from build123d import *

# Parameters (mm, degrees)
BOX_W             = 8
BOX_H             = 1
BOX_DEPTH         = 4
TUBE016_R         = 4
TUBE016_R_2       = 2.6
TUBE016_DEPTH     = 1
BOX067_W          = 8
BOX067_H          = 1
BOX067_DEPTH      = 4
TUBE019_R         = 4
TUBE019_R_2       = 2.6
TUBE019_DEPTH     = 1
BOX051_W          = 17
BOX051_H          = 8
BOX051_DEPTH      = 2
CYLINDER093_R     = 1.6
CYLINDER093_DEPTH = 8
CYLINDER094_R     = 1.6
CYLINDER094_DEPTH = 8
CYLINDER095_R     = 1.6
CYLINDER095_DEPTH = 8
CYLINDER092_R     = 1.6
CYLINDER092_DEPTH = 8
CYLINDER084_R     = 3.5
CYLINDER084_DEPTH = 2.5
BOX033_W          = 29.5
BOX033_H          = 2.5
BOX033_DEPTH      = 6
CYLINDER082_R     = 3.5
CYLINDER082_DEPTH = 2.5
BOX021_W          = 29.5
BOX021_H          = 2.5
BOX021_DEPTH      = 6
BOX022_W          = 29.5
BOX022_H          = 26
BOX022_DEPTH      = 2
BOX029_W          = 2.5
BOX029_H          = 21
BOX029_DEPTH      = 6
BOX036_W          = 2.5
BOX036_H          = 21
BOX036_DEPTH      = 6
FILLET006_R       = 2
FILLET007_R       = 2


with BuildPart() as cube:
    # Box → Box (new body)
    with BuildSketch(Plane(origin=(-4, -7, 0), x_dir=(1, 0, 0), z_dir=(0, 0, 1))):
        with Locations((4, 0.5)):
            Rectangle(BOX_W, BOX_H)
    extrude(amount=BOX_DEPTH)


with BuildPart() as cut068:
    # Tube016 → Tube016 (new body)
    with BuildSketch(Plane.XZ.offset(6)):
        Circle(TUBE016_R)
        Circle(TUBE016_R_2, mode=Mode.SUBTRACT)
    extrude(amount=TUBE016_DEPTH)

    # Cut068: cut Cube
    add(cube.part, mode=Mode.SUBTRACT)


with BuildPart() as cube067:
    # Box067 → Box067 (new body)
    with BuildSketch(Plane(origin=(-4, -34, 0), x_dir=(1, 0, 0), z_dir=(0, 0, 1))):
        with Locations((4, 0.5)):
            Rectangle(BOX067_W, BOX067_H)
    extrude(amount=BOX067_DEPTH)


with BuildPart() as cut071:
    # Tube019 → Tube019 (new body)
    with BuildSketch(Plane.XZ.offset(33)):
        Circle(TUBE019_R)
        Circle(TUBE019_R_2, mode=Mode.SUBTRACT)
    extrude(amount=TUBE019_DEPTH)

    # Cut071: cut Cube067
    add(cube067.part, mode=Mode.SUBTRACT)


with BuildPart() as cube051:
    # Box051 → Box051 (new body)
    with BuildSketch(Plane(origin=(-8.5, -49, -8), x_dir=(1, 0, 0), z_dir=(0, 0, 1))):
        with Locations((8.5, 4)):
            Rectangle(BOX051_W, BOX051_H)
    extrude(amount=BOX051_DEPTH)


with BuildPart() as cylinder093:
    # Cylinder093 → Cylinder093 (new body)
    with BuildSketch(Plane(origin=(-10, -55, 0), x_dir=(1, 0, 0), z_dir=(0, 0, 1))):
        Circle(CYLINDER093_R)
    extrude(amount=CYLINDER093_DEPTH)


with BuildPart() as cylinder094:
    # Cylinder094 → Cylinder094 (new body)
    with BuildSketch(Plane(origin=(12.5, -36, 0), x_dir=(1, 0, 0), z_dir=(0, 0, 1))):
        Circle(CYLINDER094_R)
    extrude(amount=CYLINDER094_DEPTH)


with BuildPart() as cylinder095:
    # Cylinder095 → Cylinder095 (new body)
    with BuildSketch(Plane(origin=(12.5, -55, 0), x_dir=(1, 0, 0), z_dir=(0, 0, 1))):
        Circle(CYLINDER095_R)
    extrude(amount=CYLINDER095_DEPTH)


with BuildPart() as fusion059:
    # Cylinder092 → Cylinder092 (new body)
    with BuildSketch(Plane(origin=(-10, -36, 0), x_dir=(1, 0, 0), z_dir=(0, 0, 1))):
        Circle(CYLINDER092_R)
    extrude(amount=CYLINDER092_DEPTH)

    # Fusion058: union Cylinder093, Cylinder094, Cylinder095
    add(cylinder093.part)
    add(cylinder094.part)
    add(cylinder095.part)


with BuildPart() as fusion059_1:
    # Fusion058 placement: moved
    add(fusion059.part.moved(Location((0, 0, -8))))

    # Fusion059: union Cube051
    add(cube051.part)


with BuildPart() as cylinder084:
    # Cylinder084 → Cylinder084 (new body)
    with BuildSketch(Plane.XZ.offset(55.5)):
        Circle(CYLINDER084_R)
    extrude(amount=CYLINDER084_DEPTH)


with BuildPart() as cut038:
    # Box033 → Box033 (new body)
    with BuildSketch(Plane(origin=(-13.5, -58, -6), x_dir=(1, 0, 0), z_dir=(0, 0, 1))):
        with Locations((14.75, 1.25)):
            Rectangle(BOX033_W, BOX033_H)
    extrude(amount=BOX033_DEPTH)

    # Cut038: cut Cylinder084
    add(cylinder084.part, mode=Mode.SUBTRACT)


with BuildPart() as cut038_1:
    # Cut038 placement: moved
    add(cut038.part.moved(Location((0, 23, 0))))


with BuildPart() as cylinder082:
    # Cylinder082 → Cylinder082 (new body)
    with BuildSketch(Plane.XZ.offset(55.5)):
        Circle(CYLINDER082_R)
    extrude(amount=CYLINDER082_DEPTH)


with BuildPart() as cut036:
    # Box021 → Box021 (new body)
    with BuildSketch(Plane(origin=(-13.5, -58, -6), x_dir=(1, 0, 0), z_dir=(0, 0, 1))):
        with Locations((14.75, 1.25)):
            Rectangle(BOX021_W, BOX021_H)
    extrude(amount=BOX021_DEPTH)

    # Cut036: cut Cylinder082
    add(cylinder082.part, mode=Mode.SUBTRACT)


with BuildPart() as cut036_1:
    # Cut036 placement: moved
    add(cut036.part.moved(Location((0, -0.5, 0))))


with BuildPart() as cube022:
    # Box022 → Box022 (new body)
    with BuildSketch(Plane(origin=(-13.5, -58.5, -8), x_dir=(1, 0, 0), z_dir=(0, 0, 1))):
        with Locations((14.75, 13)):
            Rectangle(BOX022_W, BOX022_H)
    extrude(amount=BOX022_DEPTH)


with BuildPart() as cube029:
    # Box029 → Box029 (new body)
    with BuildSketch(Plane(origin=(-13.5, -56, -6), x_dir=(1, 0, 0), z_dir=(0, 0, 1))):
        with Locations((1.25, 10.5)):
            Rectangle(BOX029_W, BOX029_H)
    extrude(amount=BOX029_DEPTH)


with BuildPart() as fillet007:
    # Box036 → Box036 (new body)
    with BuildSketch(Plane(origin=(13.5, -56, -6), x_dir=(1, 0, 0), z_dir=(0, 0, 1))):
        with Locations((1.25, 10.5)):
            Rectangle(BOX036_W, BOX036_H)
    extrude(amount=BOX036_DEPTH)

    # Fusion062: union Cut038, Cut036, Cube022, Cube029
    add(cut038_1.part)
    add(cut036_1.part)
    add(cube022.part)
    add(cube029.part)

    # Cut056: cut Fusion059
    add(fusion059_1.part, mode=Mode.SUBTRACT)


with BuildPart() as fillet007_1:
    # Cut056 placement: moved
    add(fillet007.part.moved(Location((0, 25.5, 0))))

    # Fusion084: union Cut068, Cut071
    add(cut068.part)
    add(cut071.part)

    # Fillet006
    fillet006_edges = [fillet007_1.edges().sort_by_distance(p)[0] for p in [
        (-13.5, -7, -3),
        (-13.5, -33, -3),
    ]]
    fillet(fillet006_edges, radius=FILLET006_R)

    # Fillet007
    fillet007_edges = [fillet007_1.edges().sort_by_distance(p)[0] for p in [
        (16, -33, -3),
        (16, -7, -3),
    ]]
    fillet(fillet007_edges, radius=FILLET007_R)


solid = fillet007_1.part
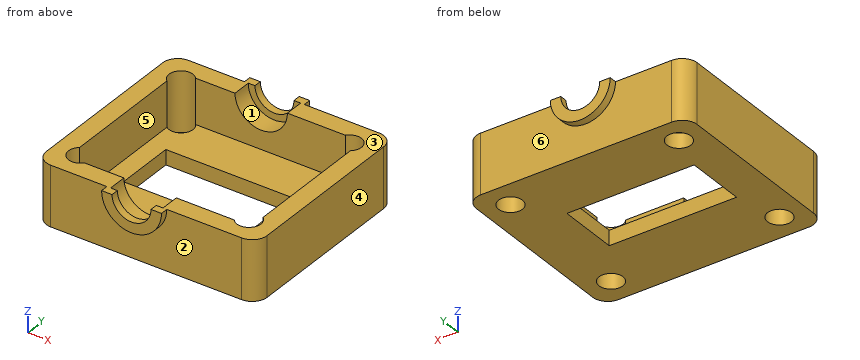
Build history of the part. All positions in model axes, mm. Face numbers are marked on the shaded views. A direction names the side the tool comes from. Give positions to 0.01 mm unless a question says otherwise; leave off trailing zeros. Order: outer loops, then holes, each group sorted by start corner. A loop starts at its lowest first (then second) coordinate and runs counter-clockwise, first axis right, second up. Notation, with made-up numbers: M 16.25,-33 L 59.25,-33 A19 ccw 59.25,-25 Z; hole C -11.5,48 d5. An arc over 180 degrees is marked long. Put each result on its own line as item: value.
Item 1: Flat gauge pins, fed straight in: pin 1 Ø2 at (x, y) = (-8.5, -30) entering from +Z; pin 2 Ø1 at (x, z) = (3, -7.5) entering from -Y; pin 3 Ø2.5 at (x, y) = (12.5, -10.5) entering from +Z; pin 4 Ø5 at (x, y) = (-6.5, -17.5) entering from +Z. Where does each tip first touch, or does it go through?
From the geometry:
pin 1: stops at z = 0
pin 2: stops at y = -33
pin 3: passes through
pin 4: stops at z = -6
Item 2: Slice it at D-D, the plane x = -10. Write the cut outline in (y, z).
From the geometry:
outline: M -33,-8 L -31.1,-8 L -31.1,0 L -33,0 Z; M -27.9,-8 L -12.1,-8 L -12.1,-6 L -27.9,-6 Z; M -8.9,-8 L -7,-8 L -7,0 L -8.9,0 Z
Item 3: Two-plate mould, pull along Y, no slides. Class the marked faces 1, 2 and 3: +Y half, -Y half, draft (parallel to the pull), parting line (faces both ways), or undercut.
From the geometry:
face 1: undercut
face 2: -Y half
face 3: draft
Item 4: 3-axis set-ups, long thin cutter, end or side, ignore diameter. For the marked faces 4, 5 and 6: which of +Z, -Z, +X, -X, +Y, -Y reach the whole face in a straight line?
From the geometry:
face 4: +Z, -Z, +X, +Y, -Y
face 5: +Z
face 6: -Z, +Y
Item 5: Slice it at C-C, the plane y = -29.5. Write the cut outline in (x, z), plus the area to 3 significant figures.
From the geometry:
outline: M -13.5,-8 L -11.6,-8 L -11.6,0 L -13.5,0 Z; M -8.4,-8 L 10.9,-8 L 10.9,-6 L -8.4,-6 Z; M 14.1,-8 L 16,-8 L 16,0 L 14.1,0 Z
area: 69.0 mm2
Item 6: Probe line 1 (Y direction, x = -10, z = -6.5); line 2 (Y direction, x = 4.5, z = -1.25); line 3 (X direction, y = -17.5, z = -2.25). List the from-to ranges inside material, lowest first. Write a range as [from, to].
From the geometry:
line 1: y = [-33, -31.1], [-27.9, -12.1], [-8.9, -7]
line 2: y = [-33, -30.5], [-9.5, -7]
line 3: x = [-13.5, -11], [13.5, 16]
Item 7: Slice it at A-A, the plane x = 0. Write the cut outline in (y, z).
From the geometry:
outline: M -34,-4 L -33,-4 L -33,-8 L -23.5,-8 L -23.5,-6 L -30.5,-6 L -30.5,-3.5 L -33,-3.5 L -33,-2.6 L -34,-2.6 Z; M -15.5,-8 L -7,-8 L -7,-4 L -6,-4 L -6,-2.6 L -7,-2.6 L -7,-3.5 L -9.5,-3.5 L -9.5,-6 L -15.5,-6 Z
Item 8: Slice it at B-B, the plane z = -6.5. Write the cut outline in (x, y), plus the area to 3 significant figures.
From the geometry:
outline: M -13.5,-31 A2 ccw -11.5,-33 L 14,-33 A2 ccw 16,-31 L 16,-9 A2 ccw 14,-7 L -11.5,-7 A2 ccw -13.5,-9 Z; hole C -10,-29.5 d3.2; hole C -10,-10.5 d3.2; hole M -8.5,-23.5 L 8.5,-23.5 L 8.5,-15.5 L -8.5,-15.5 Z; hole C 12.5,-29.5 d3.2; hole C 12.5,-10.5 d3.2
area: 595 mm2
